Can you work these out from the model? Positions are in its coordinate system, mm. A direction names the side the tool comes from. Give positions to 0.01 mm unless a question says otherwise; leave off trailing zeros. Order: outer loops, then holes, each group sorted by start corner. A loop starts at its lowest first (then second) coordinate and runs counter-clockwise, first axis right, second up. Notation, with made-up numbers: M -6.75,6.25 L 49.25,6.25 A24 cw 49.25,40.25 Z; hole C -39,18.25 d4. An arc over 180 degrees is marked long. Use one line per item in the form item = value. Start each with the question number.
1. For faces 1 (the face through (-11, 33.96, -13)), 2 (the face through (-6, 0, -19)), 3 (the face through (-10, 20.65, -13)), which set-ups out of +Z, -Z, +X, -X, +Y, -Y let a thin tool reach every point of the face, with its end or its side?
2. We'd pull the mould along Z, two halves only. Please class faces 4 (the face through (-11.32, 44.43, -19.43)), 5 (the face through (-15.43, 26.92, 8.45)), 6 (the face through (-6, 54.61, -19)): +Z half, -Z half, draft (parallel to the pull), parting line (faces both ways), or undercut.
3. I want a section at C-C, the plane y = 50. List the corners of the cut face in (x, z) for me.
4. I want a section at D-D, the plane y = 24.5. List the corners of the cut face in (x, z) for me.
5. I need wall thicknesses on L1, parallel to Y at x = -13.5, z = -13.5; L2, parallel to X at y = 28, z = -14; L3, parallel to Z at x = -10, y = 42.5. Which ranges of each line are inside material? Lowest first, please.
6. I want a section at A-A, the plane x = -12. List the corners of the cut face in (y, z) for me.
7. Will these pins go through, and if not, where does the flat tip stop? P1, Ø5, axis at y = 20, z = -17.5, coming from the -X side; P2, Ø1.5, axis at y = 38, z = -17.5, coming from the +X side; P3, Ø10, axis at x = -11, z = -12.5, coming from the -Y side.
8. I want a section at B-B, the plane z = -8.5. List the corners of the cut face in (x, y) for me, and give its area (3 significant figures).
```python
from build123d import *

# Parameters (mm, degrees)
SKETCH1_R           = 22.352
BOSS_EXTRUDE1_DEPTH = 54.61
SKETCH2_R           = 6.35
CUT_EXTRUDE1_DEPTH  = 20.6502
SKETCH3_R           = 6.35
CUT_EXTRUDE2_DEPTH  = 20.6502


with BuildPart() as part:
    # Sketch1 → Boss-Extrude1 (new body)
    with BuildSketch(Plane(origin=(0, 0, 0), x_dir=(1, 0, 0), z_dir=(0, 1, 0))):
        with Locations((-10.585213669, 13.370796213)):
            Circle(SKETCH1_R)
    extrude(amount=BOSS_EXTRUDE1_DEPTH)

    # Sketch2 → Cut-Extrude1 (cut)
    with BuildSketch(Plane(origin=(0, 54.61, 0), x_dir=(1, 0, 0), z_dir=(0, 1, 0))):
        with Locations((-10.493492602, 13.133399692)):
            Circle(SKETCH2_R)
    extrude(amount=-CUT_EXTRUDE1_DEPTH, mode=Mode.SUBTRACT)

    # Sketch3 → Cut-Extrude2 (cut)
    with BuildSketch(Plane(origin=(0, 0, 0), x_dir=(-1, 0, 0), z_dir=(0, -1, 0))):
        with Locations((10.493492678, 13.133399692)):
            Circle(SKETCH3_R)
    extrude(amount=-CUT_EXTRUDE2_DEPTH, mode=Mode.SUBTRACT)


solid = part.part
```
Check result:
q1.face_1 = +Y
q1.face_2 = +Z, -Z, +X, -X, -Y
q1.face_3 = -Y
q2.face_4 = undercut
q2.face_5 = parting line
q2.face_6 = draft
q3.outline = C -10.59,-13.37 d44.7; hole C -10.49,-13.13 d12.7
q4.outline = C -10.59,-13.37 d44.7
q5.L1 = 20.65 to 33.96
q5.L2 = -32.93 to 11.76
q5.L3 = -35.72 to -19.46, -6.8 to 8.97
q6.outline = M 0,-35.68 L 54.61,-35.68 L 54.61,-19.3 L 33.96,-19.3 L 33.96,-6.96 L 54.61,-6.96 L 54.61,8.94 L 0,8.94 L 0,-6.96 L 20.65,-6.96 L 20.65,-19.3 L 0,-19.3 Z
q7.P1 = -32.88
q7.P2 = 11.51
q7.P3 = 20.65
q8.outline = M -32.4,0 L -14.84,0 L -14.84,20.65 L -6.15,20.65 L -6.15,0 L 11.23,0 L 11.23,54.61 L -6.15,54.61 L -6.15,33.96 L -14.84,33.96 L -14.84,54.61 L -32.4,54.61 Z
q8.area = 2,020 mm2
